Geometry: see drawing. Coordinates: mm, zero at the bounding-box minimum. A direction names the side the tool comes from. Give positions to 0.01 mm unless a question says otherwise; leave off trailing zeros. Loops run counter-clockwise (first coordinate to the right, second up) from the corner with the lowest first, then second, coordinate; pieces in that order, holes last. Notation, with made-up numbers: M -11.75,3 L 35.25,3 A9 cw 35.25,18 Z; hole C 65,67 d7. An arc over 180 degrees is marked long. Answer in a Markdown table with one row per item.
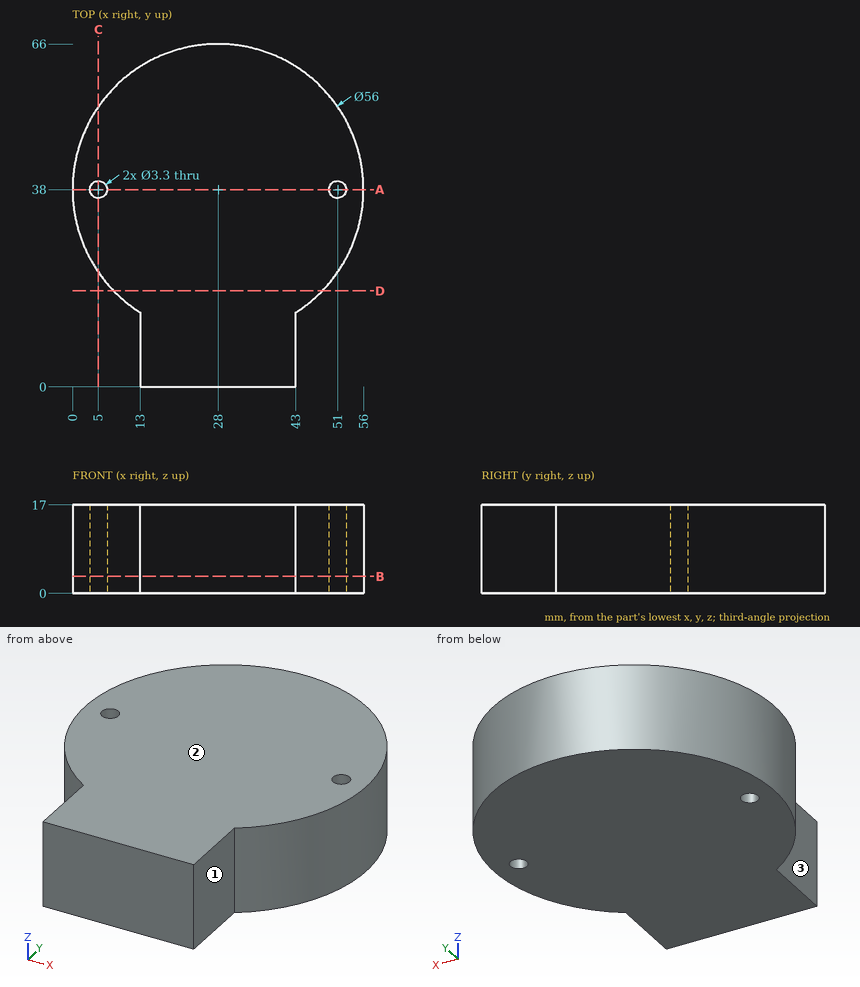
1) Section C-C, the plane x = 5. Return loops of the section in (y, z), then the cut area to 3 significant figures.
Reply:
| item | result |
|---|---|
| outline | M 22.03,0 L 36.35,0 L 36.35,17 L 22.03,17 Z; M 39.65,0 L 53.97,0 L 53.97,17 L 39.65,17 Z |
| area | 487 mm² |
2) Section B-B, the plane z = 3.25. Return loops of the section in (x, y), then the cut area to 3 significant figures.
Reply:
| item | result |
|---|---|
| outline | M 13,0 L 43,0 L 43,14.36 A28 ccw long 13,14.36 Z; hole C 5,38 d3.3; hole C 51,38 d3.3 |
| area | 2,790 mm² |
3) Pin query (flat end, axial travel): pin 1 Ø10 at (x, z) = (10.5, 8.5) entering from +Y; pin 2 Ø1.5 at (y, z) = (26, 12.5) entering from +X; pin 3 Ø1.5 at (y, z) = (29, 3.5) entering from +X. Return the tip coordinate at first contact, or that it passes through.
Reply:
| item | result |
|---|---|
| pin 1 | stops at y = 63.05 |
| pin 2 | stops at x = 53.64 |
| pin 3 | stops at x = 54.76 |
4) Section A-A, the plane y = 38. Return loops of the section in (x, z), then the cut area to 3 significant figures.
Reply:
| item | result |
|---|---|
| outline | M 0,0 L 3.35,0 L 3.35,17 L 0,17 Z; M 6.65,0 L 49.35,0 L 49.35,17 L 6.65,17 Z; M 52.65,0 L 56,0 L 56,17 L 52.65,17 Z |
| area | 840 mm² |
5) Set-up query: the marked faces 1, 2 and 3. Return all of +Z, -Z, +X, -X, +Y, -Y with unobstructed straight access to the full face (end or side cutting, diameter ignored); none if empty.
Reply:
| item | result |
|---|---|
| face 1 | +Z, -Z, +X, -Y |
| face 2 | +Z, +X, -X, +Y, -Y |
| face 3 | +Z, -Z, -X, -Y |
6) Section D-D, the plane y = 18.5. Return loops of the section in (x, z), then the cut area to 3 significant figures.
Reply:
| item | result |
|---|---|
| outline | M 7.91,0 L 48.09,0 L 48.09,17 L 7.91,17 Z |
| area | 683 mm² |
7) Material intervals for L1, parallel to X at y = 39.5, z = 7.75; L2, parallel to Y at x = 51, z = 5; L3, parallel to Y at x = 4.5, z = 7, sorted ascending.
Reply:
| item | result |
|---|---|
| L1 | x = 0.04 to 4.31, 5.69 to 50.31, 51.69 to 55.96 |
| L2 | y = 22.03 to 36.35, 39.65 to 53.97 |
| L3 | y = 22.78 to 36.43, 39.57 to 53.22 |
